Check sheet for the modelled part. Datum: model origin and axes. Units: mm. Face numbers are marked on the shaded views. A direction names the side the tool comes from. Round coordinates to 2 decimals unless told otherwise and drop trailing zeros. Order: outer loops, then holes, each group sorted by start corner. A loop starts at its lowest first (then second) coordinate and runs counter-clockwise, first axis right, second up. Notation, with made-up numbers: (2, 77) -> (40, 77) arc R23 cw to (40, 85) -> close; hole circle Ø10 at (20.25, 11.25). An arc over 180 degrees is marked (long way). Answer in a Markdown table with one row per item. Add a question column.
1. Sectioned sample at A-A, the plane z = 0. Record the boundary of the cut face in (x, y).
2. Sectioned sample at B-B, the plane x = 0. Record the boundary of the cut face in (y, z), then the cut area to 3 significant figures.
3. Depth check by flat-ended pin: P1, Ø4, axis at x = 17.5, y = 3, coming from the +Z side; P2, Ø6.5, axis at x = 20, y = 7.5, coming from the -Z side; P3, Ø5, axis at x = -12, y = 5, coming from the -Z side. Enter the tip coordinate at first touch or a pass-through.
4. Draft check along X on the marked faces 1, 2 and 3. Enter one of: +X half, -X half, draft (parallel to the pull), parting line (faces both ways), or undercut.
5. Access from +Z, -Z, +X, -X, +Y, -Y to the whole of each face (thin tool, end or side, straight path). Record for the marked faces 4, 5, 6 and 7.
6. Material ranges on L1, parallel to Z at x = 0, y = 3.75; L2, parallel to Z at x = -22, y = 5; L3, parallel to X at y = 3.5, z = 11, recorded low to high. Write a range as from..to.
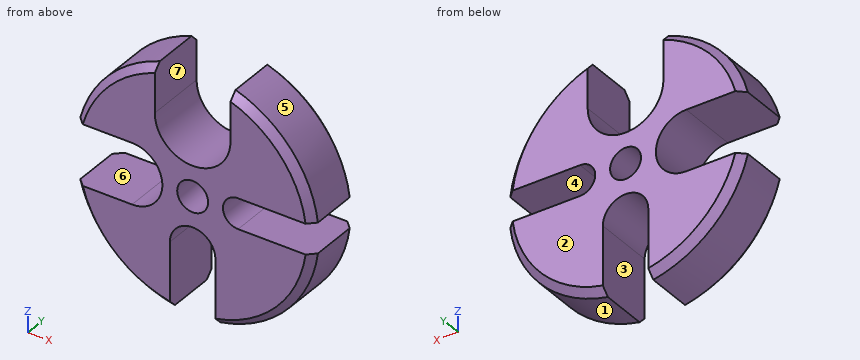
```python
from build123d import *

# Parameters (mm, degrees)
SKETCH1_R           = 25.4
BOSS_EXTRUDE1_DEPTH = 12.7
HOLE1_D             = 6.477
CUT_EXTRUDE4_DEPTH  = 39.1
CIRPATTERN1_DEPTH   = 12.7
CHAMFER1_SIZE       = 1.524


# Read off the part's stored shape, not the designer's step: CirPattern1
with BuildPart() as part:
    # Sketch1 → Boss-Extrude1 (new body)
    with BuildSketch(Plane(origin=(0, 0, 0), x_dir=(1, 0, 0), z_dir=(0, 1, 0))):
        with Locations(Location((0, 0, 0), (0, 0, 270))):
            Circle(SKETCH1_R)
    extrude(amount=BOSS_EXTRUDE1_DEPTH)

    # Hole1 (through all)
    with Locations(Plane(origin=(0, 12.7, 0), x_dir=(1, 0, 0), z_dir=(0, 1, 0))):
        with Locations((0, 0)):
            Hole(HOLE1_D / 2)

    # Sketch4 → Cut-Extrude4 (cut, symmetric)
    with BuildSketch(Plane(origin=(0, 12.7, 0), x_dir=(1, 0, 0), z_dir=(0, 1, 0))):
        with BuildLine():
            Line((-4.7625, 152.335221274), (-4.7625, 24.949520912))
            Line((-4.7625, 24.949520912), (-4.7625, 11.0998))
            ThreePointArc((-4.7625, 11.0998), (0, 6.3373), (4.7625, 11.0998))
            Line((4.7625, 11.0998), (4.7625, 24.949520912))
            Line((4.7625, 24.949520912), (4.7625, 152.335221274))
            Line((4.7625, 152.335221274), (4.7625, 407.106621997))
            Line((4.7625, 407.106621997), (-4.7625, 407.106621997))
            Line((-4.7625, 407.106621997), (-4.7625, 152.335221274))
        make_face()
    extrude(amount=CUT_EXTRUDE4_DEPTH, both=True, mode=Mode.SUBTRACT)

    # CirPattern1 outline → CirPattern1 (cut)
    with BuildSketch(Plane(origin=(0, 0, 0), x_dir=(1, 0, 0), z_dir=(0, 1, 0))):
        with BuildLine():
            ThreePointArc((-24.593444248, 6.35), (-25.4, 0), (-24.593444248, -6.35))
            Line((-24.593444248, -6.35), (-12.7, -6.35))
            ThreePointArc((-12.7, -6.35), (-6.35, 0), (-12.7, 6.35))
            Line((-12.7, 6.35), (-24.593444248, 6.35))
        make_face()
        with BuildLine():
            Line((9.525, -3.175), (25.200781238, -3.175))
            ThreePointArc((25.200781238, -3.175), (25.4, 0), (25.200781238, 3.175))
            Line((25.200781238, 3.175), (9.525, 3.175))
            ThreePointArc((9.525, 3.175), (6.35, 0), (9.525, -3.175))
        make_face()
        with BuildLine():
            Line((-7.9375, -14.2748), (-7.9375, -24.127911094))
            ThreePointArc((-7.9375, -24.127911094), (0, -25.4), (7.9375, -24.127911094))
            Line((7.9375, -24.127911094), (7.9375, -14.2748))
            ThreePointArc((7.9375, -14.2748), (0, -6.3373), (-7.9375, -14.2748))
        make_face()
    extrude(amount=CIRPATTERN1_DEPTH, mode=Mode.SUBTRACT)

    # Chamfer1
    chamfer1_edges = [part.edges().sort_by_distance(p)[0] for p in [
        (-17.37608731, 0, -18.526510459),
        (-17.37608731, 12.7, -18.526510459),
        (-18.535887196, 0, 17.366084356),
        (-18.535887196, 12.7, 17.366084356),
        (19.603380874, 0, 16.151391839),
        (19.603380874, 12.7, 16.151391839),
        (18.519773105, 0, -17.383267936),
        (18.519773105, 12.7, -17.383267936),
    ]]
    chamfer(chamfer1_edges, length=CHAMFER1_SIZE)


solid = part.part
```
Answer key:
| question | item | result |
|---|---|---|
| 1 | outline | (-6.35, 0) -> (-3.24, 0) -> (-3.24, 12.7) -> (-6.35, 12.7) -> close; (3.24, 0) -> (6.35, 0) -> (6.35, 12.7) -> (3.24, 12.7) -> close |
| 2 | outline | (0, -6.34) -> (12.7, -6.34) -> (12.7, -3.24) -> (0, -3.24) -> close; (0, 3.24) -> (12.7, 3.24) -> (12.7, 6.34) -> (0, 6.34) -> close |
| 2 | area | 78.7 mm² |
| 3 | P1 | stops at z = 20.12 |
| 3 | P2 | stops at z = -19.09 |
| 3 | P3 | stops at z = -23.56 |
| 4 | face 1 | +X half |
| 4 | face 2 | draft |
| 4 | face 3 | undercut |
| 5 | face 4 | +X, +Y, -Y |
| 5 | face 5 | +Z, +X, +Y, -Y |
| 5 | face 6 | -X, +Y, -Y |
| 5 | face 7 | +Z, +Y, -Y |
| 6 | L1 | z = -6.34..-3.24, 3.24..6.34 |
| 6 | L2 | z = -12.69..-6.35, 6.35..12.69 |
| 6 | L3 | x = -22.89..-7.23, 7.23..22.89 |
